Can you work these out from the model? Positions are in its coordinate system, mm. Give positions to 0.01 mm unless a question says otherwise; leave off trailing zeros. Loops run counter-clockwise (first coordinate to the right, second up) from the corner with the lowest first, then second, coordinate; pieces in that order, holes last. Notation, with made-up numbers: (32, 78) - (67, 78) arc R19 cw to (67, 90) - close; hole circle Ø6 at (82.5, 80). An arc over 180 degrees is marked (long way). Answer as a JSON object with one key per item and string values.
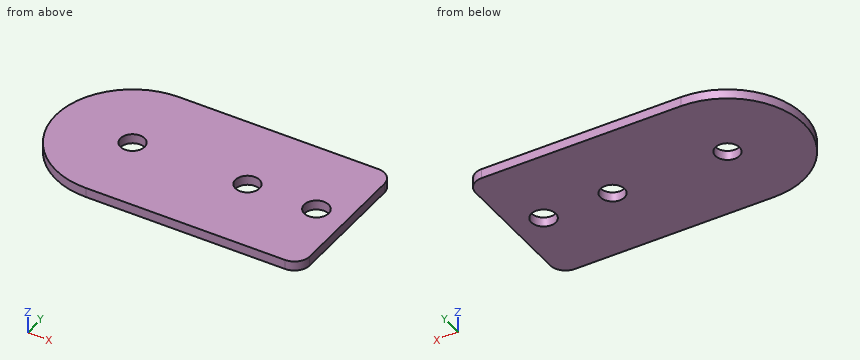
```python
from build123d import *

# Parameters (mm, degrees)
SKETCH1_R           = 2
SKETCH1_R_2         = 2.032
BOSS_EXTRUDE1_DEPTH = 1.5875
FILLET1_R           = 2.54


with BuildPart() as part:
    # Sketch1 → Boss-Extrude1 (new body)
    with BuildSketch(Plane.XY):
        with BuildLine():
            Line((0, -12.7), (35.56, -12.7))
            Line((35.56, -12.7), (35.56, 12.7))
            Line((35.56, 12.7), (0, 12.7))
            ThreePointArc((0, 12.7), (-12.7, 0), (0, -12.7))
        make_face()
        Circle(SKETCH1_R, mode=Mode.SUBTRACT)
        with Locations((19.05, 0)):
            Circle(SKETCH1_R, mode=Mode.SUBTRACT)
        with Locations((30.48, 0)):
            Circle(SKETCH1_R_2, mode=Mode.SUBTRACT)
    extrude(amount=BOSS_EXTRUDE1_DEPTH)

    # Fillet1
    fillet1_edges = [part.edges().sort_by_distance(p)[0] for p in [
        (35.56, 12.7, 0.79375),
        (35.56, -12.7, 0.79375),
    ]]
    fillet(fillet1_edges, radius=FILLET1_R)


solid = part.part
```
1) Imagine slicing it at C-C on z = 0.95. Write out the boundary of the cut face in (x, y), and give its area (3 significant figures).
Check sheet entries:
{"outline": "(0, -12.7) - (33.02, -12.7) arc R2.54 ccw to (35.56, -10.16) - (35.56, 10.16) arc R2.54 ccw to (33.02, 12.7) - (0, 12.7) arc R12.7 ccw to start; hole circle Ø4 at (0, 0); hole circle Ø4 at (19.05, 0); hole circle Ø4.06 at (30.48, 0)", "area": "1,120 mm2"}
2) I need wall thicknesses on L1, parallel to Y at x = 0, z = 0.7; L2, parallel to Y at x = 17.5, z = 0.4; L3, parallel to X at y = -3.5, z = 0.9. Which ranges of each line are inside material? Lowest first, please.
Check sheet entries:
{"L1": "-12.7 to -2, 2 to 12.7", "L2": "-12.7 to -1.26, 1.26 to 12.7", "L3": "-12.21 to 35.56"}
3) Imagine slicing it at A-A on x = 30.48. Write out the boundary of the cut face in (y, z).
Check sheet entries:
{"outline": "(-12.7, 0) - (-2.03, 0) - (-2.03, 1.59) - (-12.7, 1.59) - close; (2.03, 0) - (12.7, 0) - (12.7, 1.59) - (2.03, 1.59) - close"}
4) Imagine slicing it at B-B on y = 0. Write out the boundary of the cut face in (x, z).
Check sheet entries:
{"outline": "(-12.7, 0) - (-2, 0) - (-2, 1.59) - (-12.7, 1.59) - close; (2, 0) - (17.05, 0) - (17.05, 1.59) - (2, 1.59) - close; (21.05, 0) - (28.45, 0) - (28.45, 1.59) - (21.05, 1.59) - close; (32.51, 0) - (35.56, 0) - (35.56, 1.59) - (32.51, 1.59) - close"}
5) Imagine slicing it at D-D on x = 19.05. Write out the boundary of the cut face in (y, z), and give its area (3 significant figures).
Check sheet entries:
{"outline": "(-12.7, 0) - (-2, 0) - (-2, 1.59) - (-12.7, 1.59) - close; (2, 0) - (12.7, 0) - (12.7, 1.59) - (2, 1.59) - close", "area": "34.0 mm2"}
